Autodesk Inventor part; units mm, degrees
ref_plane "YZ Plane" through (0, 0, 0) normal (1, 0, 0) x (0, 1, 0)
ref_plane "XZ Plane" through (0, 0, 0) normal (0, 1, 0) x (-1, 0, 0)
ref_plane "XY Plane" through (0, 0, 0) normal (0, 0, 1) x (1, 0, 0)
sketch "Sketch1" plane through (0, 0, 0) normal (0, 0, 1) x (1, 0, 0)
  line L0 (0, 0) -> (29.6, 0) construction
  line L1 (0, -12.7) -> (29.6, -12.7)
  line L2 (29.6, 12.7) -> (0, 12.7)
  arc A0 (0, 12.7) -> (0, -12.7) centre (0, 0) ccw
  arc A1 (29.6, -12.7) -> (29.6, 12.7) centre (29.6, 0) ccw
  circle A2 centre (0, 0) radius 2.65
  circle A3 centre (29.6, 0) radius 2.65
  point P0 (14.8, 0)
  dimension "d0" = 29.6
  dimension "d1" = 5.3
  dimension "d2" = 5.3
  dimension "d9" = 25.4
extrude "Extrusion1" add sketch "Sketch1" along normal blind 29.425
sketch "Sketch2" plane through (0, 0, 29.425) normal (0, 0, 1) x (1, 0, 0)
  circle A0 centre (0, 0) radius 2.65
  circle A1 centre (29.6, 0) radius 2.65
  circle A2 centre (0, 0) radius 6
  circle A3 centre (29.6, 0) radius 6
  dimension "d6" = 12
extrude "Extrusion2" cut sketch "Sketch2" against normal blind 5
chamfer "Chamfer1" distance 3 angle 45 4 edges at (14.8, 12.7, 29.425) (-12.7, 0, 29.425) (14.8, -12.7, 29.425) (42.3, 0, 29.425)
properties part number "Tope" material "ABS Plastic"
Geometry: final body of the model. Coordinates: model frame, mm. A direction names the side the tool comes from. Coordinates: 2 decimals unless noted, no trailing zeros. Order: outer loops, then holes, each group sorted by start corner. A loop starts at its lowest first (then second) coordinate and runs counter-clockwise, first axis right, second up.
(1) First-contact query: pin 1 (14 mm diameter, centred on x = 0, y = 0, fed in from +Z) (3 decimals). Flat tip, straight axial feed; report the tip coordinate or a pass-through.
(2) Section query B-B (z = 3.5). Return the cut outline in (x, y).
(3) Section query A-A (y = 0). Return the cut outline in (x, z) (3 decimals).
(4) Draft query along X for faces 1 (the face through (-6, 0, 27)), 2 (the face through (14.593, 11.179, 27.946)), 3 (the face through (-12.697, -0.279, 13.028)), 4 (the face through (42.297, 0.279, 13.028)). Return one class per face: pulls with the +X half, pulls with the -X half, needs draft (parallel to the pull), parting line crosses it, or undercut.
(5) Section query C-C (x = 28.5). Return the cut outline in (y, z) (3 decimals), plus the area to 3 significant figures.
(6) Access query for faces 5 (the face through (14, 0, 29.425)), 6 (the face through (31, -3, 24.425)). Directions: +Z, -Z, +X, -X, +Y, -Y. A direction counts if a zero-diameter tool reaches every point of the face in a straight line with its end or side. Return the directions, or none.
(7) Material intervals for probe 1 along Y at (x, z) = (0, 20.75); probe 2 along X at (y, z) = (0.75, 24.25); probe 3 along Y at (x, z) = (0, 27.5) (3 decimals), sorted ascending.
Solution:
1. pin 1: stops at z = 29.425
2. outline: (0, -12.7) - (29.6, -12.7) arc R12.7 ccw to (29.6, 12.7) - (0, 12.7) arc R12.7 ccw to start; hole circle Ø5.3 at (0, 0); hole circle Ø5.3 at (29.6, 0)
3. outline: (-12.7, 0) - (-2.65, 0) - (-2.65, 24.425) - (-6, 24.425) - (-6, 29.425) - (-9.7, 29.425) - (-12.7, 26.425) - close; (2.65, 0) - (26.95, 0) - (26.95, 24.425) - (23.6, 24.425) - (23.6, 29.425) - (6, 29.425) - (6, 24.425) - (2.65, 24.425) - close; (32.25, 0) - (42.3, 0) - (42.3, 26.425) - (39.3, 29.425) - (35.6, 29.425) - (35.6, 24.425) - (32.25, 24.425) - close
4. face 1: undercut
4. face 2: needs draft
4. face 3: pulls with the -X half
4. face 4: pulls with the +X half
5. outline: (-12.7, 0) - (-2.411, 0) - (-2.411, 24.425) - (-5.898, 24.425) - (-5.898, 29.425) - (-9.7, 29.425) - (-12.7, 26.425) - close; (2.411, 0) - (12.7, 0) - (12.7, 26.425) - (9.7, 29.425) - (5.898, 29.425) - (5.898, 24.425) - (2.411, 24.425) - close
5. area: 562 mm2
6. face 5: +Z, +X, -X, +Y, -Y
6. face 6: +Z
7. probe 1: y = -12.7 to -2.65, 2.65 to 12.7
7. probe 2: x = -12.68 to -2.54, 2.54 to 27.06, 32.14 to 42.28
7. probe 3: y = -11.625 to -6, 6 to 11.625
